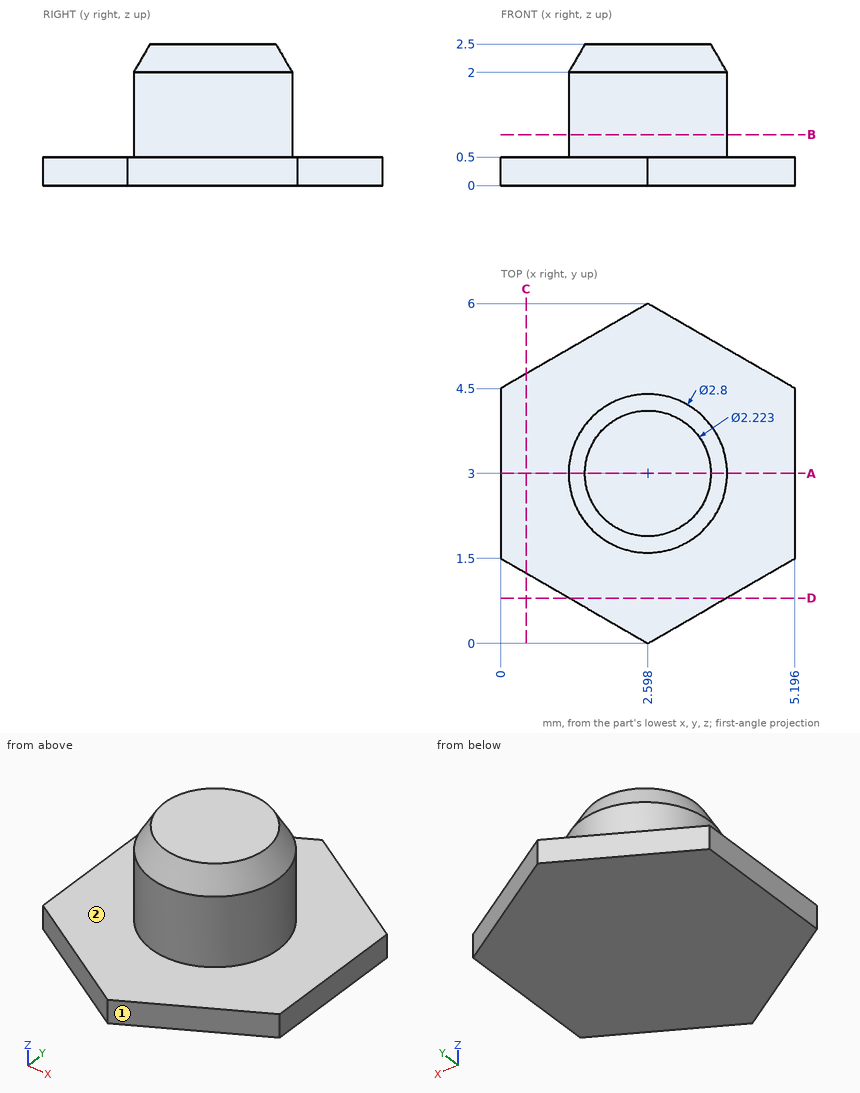
Study the drawing (mm; zero at the part's minimum x, y, z) and answer. A direction names the side the tool comes from. Give positions to 0.01 mm unless a question says otherwise; leave off trailing zeros. Write each loop counter-clockwise with the first axis right and the second up, starting at its lowest first coordinate (ties: lowest second). Pieces come first, ordered by that corner, then holes.
Item 1: A flat-ended cylindrical pin translates along its axis: P1, Ø1.5, axis at y = 4.5, z = 1.5, coming from the -X side (1 decimal). Find the tip coordinate at first contact, or state that the pin passes through.
Item 2: Section D-D, the plane y = 0.8 is taken. Write down the section's boundary in (x, z).
Item 3: Which of the six approach directions +Z, -Z, +X, -X, +Y, -Y give full straight-line access (tool end or side, diameter ignored) to the marked faces 1 and 2?
Item 4: Section C-C, the plane x = 0.45 is taken. Write down the section's boundary in (y, z).
Item 5: Section A-A, the plane y = 3 is taken. Write down the section's boundary in (x, z).
Item 6: Section B-B, the plane z = 0.9 is taken. Write down the section's boundary in (x, y).
Item 7: Find the intervals of material crossed by line 1 along Z through (x, y) = (4.5, 4.3); line 2 along Y through (x, z) = (2.65, 1.75); line 3 along X through (y, z) = (2.7, 1.45) (1 decimal), in increasing order.
Completed:
1. P1: stops at x = 1.4
2. outline: (1.21, 0) - (3.98, 0) - (3.98, 0.5) - (1.21, 0.5) - close
3. face 1: +Z, -Z, +X, -Y
3. face 2: +Z
4. outline: (1.24, 0) - (4.76, 0) - (4.76, 0.5) - (1.24, 0.5) - close
5. outline: (0, 0) - (5.2, 0) - (5.2, 0.5) - (4, 0.5) - (4, 2) - (3.71, 2.5) - (1.49, 2.5) - (1.2, 2) - (1.2, 0.5) - (0, 0.5) - close
6. outline: circle Ø2.8 at (2.6, 3)
7. line 1: z = 0 to 0.5
7. line 2: y = 1.6 to 4.4
7. line 3: x = 1.2 to 4
